Source: CAD feature listing. Evaluate the final solid. Frame: model axes, mm. Give positions to 0.01 mm unless a question says otherwise; leave off trailing zeros. Order: outer loops, then holes, each group sorted by start corner. A loop starts at its lowest first (then second) coordinate and runs counter-clockwise, first axis right, second up. Notation, with made-up numbers: (41.25, 66.5) - (79.25, 66.5) arc R26 cw to (79.25, 88.5) - close; hole circle Ø2 at (-38, 21). An arc over 180 degrees is marked (long way). Answer as CSV lines item,"result".
```python
from build123d import *

# Parameters (mm, degrees)
SKETCH4_W = 0.2
SKETCH4_H = 0.2


with BuildPart() as part:
    # Sweep2: sweep along a path in Sketch3
    with BuildLine(Plane.XY) as sweep2_path:
        Line((35, 10), (-35, 10))
        Line((-35, 10), (-35, -10))
        Line((-35, -10), (35, -10))
        Line((35, -10), (35, 8))
        Line((35, 8), (-33, 8))
        Line((-33, 8), (-33, -8))
        Line((-33, -8), (33, -8))
        Line((33, -8), (33, 6))
        Line((33, 6), (-31, 6))
        Line((-31, 6), (-31, -6))
        Line((-31, -6), (31, -6))
        Line((31, -6), (31, 4))
        Line((31, 4), (-29, 4))
        Line((-29, 4), (-29, -4))
        Line((-29, -4), (29, -4))
        Line((29, -4), (29, 2))
        Line((29, 2), (-27, 2))
        Line((-27, 2), (-27, -2))
        Line((-27, -2), (27, -2))
        Line((27, -2), (27, 0))
        Line((27, 0), (-25, 0))
    # Sketch4 → Sweep2 (sweep)
    with BuildSketch(Plane(origin=(0, 0, 0), x_dir=(0, 0, -1), z_dir=(1, 0, 0))):
        Rectangle(SKETCH4_W, SKETCH4_H)
    sweep(path=sweep2_path.line, transition=Transition.RIGHT)


solid = part.part
```
(1) Cut plane A-A (y = -7). Return loops of the section in (x, z).
Completed:
outline,"(-35.1, -0.1) - (-34.9, -0.1) - (-34.9, 0.1) - (-35.1, 0.1) - close; (-33.1, -0.1) - (-32.9, -0.1) - (-32.9, 0.1) - (-33.1, 0.1) - close; (32.9, -0.1) - (33.1, -0.1) - (33.1, 0.1) - (32.9, 0.1) - close; (34.9, -0.1) - (35.1, -0.1) - (35.1, 0.1) - (34.9, 0.1) - close"
(2) Cut plane B-B (x = -11). Give the number of separate pieces and of enclosed holes in the cut face, then the cut area to 3 significant figures.
Completed:
separate pieces,"11"
enclosed holes,"0"
area,"0.440 mm²"
(3) Ray query, line 1 (X direction, y = -7.25, z = 0.05); line 2 (X direction, y = -8, z = 0.05). Return the intervals inside material, ascending. Write a range as from..to.
Completed:
line 1,"-35.1..-34.9, -33.1..-32.9, 32.9..33.1, 34.9..35.1"
line 2,"-35.1..-34.9, -33.1..33.1, 34.9..35.1"
